```python
from build123d import *

# Parameters (mm, degrees)
F0_W     = 127
F0_H     = 127
F0_R     = 3.175
F1_DEPTH = 25.4


with BuildPart() as f1:
    # F0 (on Front) → F1 (new body)
    with BuildSketch(Plane.XZ):
        Rectangle(F0_W, F0_H)
        with Locations((-25.4, -43.994091)):
            Circle(F0_R, mode=Mode.SUBTRACT)
        with Locations((-43.994091, -25.4)):
            Circle(F0_R, mode=Mode.SUBTRACT)
        with Locations((0, -50.8)):
            Circle(F0_R, mode=Mode.SUBTRACT)
        with Locations((25.4, -43.994091)):
            Circle(F0_R, mode=Mode.SUBTRACT)
        with Locations((43.994091, -25.4)):
            Circle(F0_R, mode=Mode.SUBTRACT)
        with Locations((-50.8, 0)):
            Circle(F0_R, mode=Mode.SUBTRACT)
        with Locations((-43.994091, 25.4)):
            Circle(F0_R, mode=Mode.SUBTRACT)
        with Locations((-25.4, 43.994091)):
            Circle(F0_R, mode=Mode.SUBTRACT)
        Circle(F0_R, mode=Mode.SUBTRACT)
        with Locations((50.8, 0)):
            Circle(F0_R, mode=Mode.SUBTRACT)
        with Locations((43.994091, 25.4)):
            Circle(F0_R, mode=Mode.SUBTRACT)
        with Locations((25.4, 43.994091)):
            Circle(F0_R, mode=Mode.SUBTRACT)
        with Locations((0, 50.8)):
            Circle(F0_R, mode=Mode.SUBTRACT)
    extrude(amount=F1_DEPTH)


solid = f1.part
```
Model file for the job. Use its own axes, mm. Coordinates: 2 decimals unless noted, no trailing zeros. Write each loop counter-clockwise with the first axis right and the second up, starting at its lowest first coordinate (ties: lowest second). Pieces come first, ordered by that corner, then holes. Notation, with made-up numbers: (17.25, 82.25) - (24.25, 82.25) arc R11 ccw to (24.25, 98.25) - close; hole circle Ø7 at (4, 75.5). An arc over 180 degrees is marked (long way). One line per question, with ' | ' between items. Start each with the question number.
Q1. Drill centre lines: line 1 (Z direction, x = -25, y = -17); line 2 (X direction, y = -3, z = 42); line 3 (Z direction, x = -51, y = -13.5). Where is each one in solid material? Low to high. Write a range as [from, to].
Q2. Pull direction Z, two halves, no side cores. Call faces 1 (the face through (63.5, -13, -1)), 2 (the face through (-42.29, -12.52, 28.08)), 3 (the face through (-1, -13, 63.5)): pulls with the +Z half, pulls with the -Z half, needs draft (parallel to the pull), parting line crosses it, or undercut.
Q3. Cut at A-A, the plane z = -25.4. List the corners of the cut face in (x, y).
Q4. Cut at B-B, the plane x = -25.4. List the corners of the cut face in (y, z), then the cut area to 3 significant figures.
Q5. Cut at D-D, the plane y = -10.5. Give the number of separate pieces and of enclosed holes in the cut face, then the cut area to 3 significant figures.
Q6. Cut at C-C, the plane z = -50.8. List the corners of the cut face in (x, y) (3 decimals).
Answer below:
1) line 1: [-63.5, -47.14], [-40.84, 40.84], [47.14, 63.5] | line 2: [-63.5, -27.87], [-22.93, 22.93], [27.87, 63.5] | line 3: [-63.5, -3.17], [3.17, 63.5]
2) face 1: needs draft | face 2: undercut | face 3: pulls with the +Z half
3) outline: (-63.5, -25.4) - (-47.17, -25.4) - (-47.17, 0) - (-63.5, 0) - close; (-40.82, -25.4) - (40.82, -25.4) - (40.82, 0) - (-40.82, 0) - close; (47.17, -25.4) - (63.5, -25.4) - (63.5, 0) - (47.17, 0) - close
4) outline: (-25.4, -63.5) - (0, -63.5) - (0, -47.17) - (-25.4, -47.17) - close; (-25.4, -40.82) - (0, -40.82) - (0, 40.82) - (-25.4, 40.82) - close; (-25.4, 47.17) - (0, 47.17) - (0, 63.5) - (-25.4, 63.5) - close | area: 2,900 mm^2
5) separate pieces: 1 | enclosed holes: 13 | area: 15,700 mm^2
6) outline: (-63.5, -25.4) - (-3.175, -25.4) - (-3.175, 0) - (-63.5, 0) - close; (3.175, -25.4) - (63.5, -25.4) - (63.5, 0) - (3.175, 0) - close
